from build123d import *

# Parameters (mm, degrees)
SKETCH1_R                 = 15.24
SKETCH1_R_2               = 6.35
BOSS_EXTRUDE1_DEPTH       = 6.35
F_4_CLEARANCE_HOLE1_D     = 2.9464
F_4_CLEARANCE_HOLE1_DEPTH = 6.35
BOSS_EXTRUDE2_DEPTH       = 6.35
CIRPATTERN1_COUNT         = 4


with BuildPart() as part:
    # Sketch1 → Boss-Extrude1 (new body)
    with BuildSketch(Plane(origin=(0, 0, 0), x_dir=(1, 0, 0), z_dir=(0, 1, 0))):
        Circle(SKETCH1_R)
        Circle(SKETCH1_R_2, mode=Mode.SUBTRACT)
    extrude(amount=BOSS_EXTRUDE1_DEPTH)

    # #4 Clearance Hole1
    with Locations(Plane(origin=(-8.015495471, 6.35, -5.066061758), x_dir=(1, 0, 0), z_dir=(0, 1, 0))):
        with Locations((8.015495471, 7.633938242), (-4.684504529, -5.066061758), (20.715495471, -5.066061758), (8.015495471, -17.766061758)):
            Hole(F_4_CLEARANCE_HOLE1_D / 2, depth=F_4_CLEARANCE_HOLE1_DEPTH)

    # Sketch7 → Boss-Extrude2 (add)
    with BuildSketch(Plane(origin=(0, 6.35, 0), x_dir=(1, 0, 0), z_dir=(0, 1, 0))):
        with BuildLine():
            ThreePointArc((-6.234328974, 13.9065), (0, 19.05), (6.234328974, 13.9065))
            ThreePointArc((6.234328974, 13.9065), (0, 15.24), (-6.234328974, 13.9065))
        make_face()
    boss_extrude2 = extrude(amount=-BOSS_EXTRUDE2_DEPTH)

    # CirPattern1: Boss-Extrude2 ×4 about axis
    cirpattern1_axis = Axis((0, 0, 0), (0, 1, 0))
    for i in range(1, CIRPATTERN1_COUNT):
        add(boss_extrude2.rotate(cirpattern1_axis, i * 360 / CIRPATTERN1_COUNT))


solid = part.part
Input: part model. Units: mm. Frame: model coordinates. Coordinates: 2 decimals unless noted, no trailing zeros. Order: outer loops, then holes, each group sorted by start corner. A loop starts at its lowest first (then second) coordinate and runs counter-clockwise, first axis right, second up. Notation, with made-up numbers: M 8.25,-15.5 L 45.25,-15.5 A23 cw 45.25,8.5 Z; hole C 59.5,-18 d2. An arc over 180 degrees is marked long. One line per question, with ' | ' between items.
Item 1: Pin query (flat end, axial travel): pin 1 (1.5 mm diameter, centred on x = -8, y = 5.5, fed in from -Z); pin 2 (1.8 mm diameter, centred on x = 12.7, z = 0, fed in from -Y). Return the tip coordinate at first contact, or that it passes through.
Geometry results:
pin 1: stops at z = -13.41 | pin 2: passes through
Item 2: Ray query, line 1 along Z through (x, y) = (3, 4); line 2 along X through (y, z) = (4.5, 12.7). Return the intervals inside material, ascending.
Geometry results:
line 1: z = -18.3 to -5.6, 5.6 to 18.3 | line 2: x = -8.42 to -1.47, 1.47 to 8.42
Item 3: Draft query along Z for faces 1 (the cylindrical face through (0.32, 3.13, -11.26)), 2 (the cylindrical face through (10.72, 3.13, 10.83)), 3 (the cylindrical face through (-19.05, 3.22, 0.12)). Return one class per face: released by +Z, released by -Z, zero draft, split by the parting line, or undercut.
Geometry results:
face 1: undercut | face 2: released by +Z | face 3: split by the parting line
Item 4: Section D-D (x = -12.7). Output: boundary loops of the cut face in (y, z), then the cut area to 3 significant figures.
Geometry results:
outline: M 0,-8.42 L 6.35,-8.42 L 6.35,-1.47 L 0,-1.47 Z; M 0,1.47 L 6.35,1.47 L 6.35,8.42 L 0,8.42 Z | area: 88.3 mm^2
Item 5: Section B-B (z = 0). Output: boundary loops of the cut face in (x, y), then the cut area to 3 significant figures.
Geometry results:
outline: M -19.05,0 L -14.17,0 L -14.17,6.35 L -19.05,6.35 Z; M -11.23,0 L -6.35,0 L -6.35,6.35 L -11.23,6.35 Z; M 6.35,0 L 11.23,0 L 11.23,6.35 L 6.35,6.35 Z; M 14.17,0 L 19.05,0 L 19.05,6.35 L 14.17,6.35 Z | area: 124 mm^2
Item 6: Section C-C (z = 4). Output: boundary loops of the cut face in (x, y), then the cut area to 3 significant figures.
Geometry results:
outline: M -17.63,0 L -4.93,0 L -4.93,6.35 L -17.63,6.35 Z; M 4.93,0 L 17.63,0 L 17.63,6.35 L 4.93,6.35 Z | area: 161 mm^2
Item 7: Section A-A (x = 0). Output: boundary loops of the cut face in (y, z).
Geometry results:
outline: M 0,-19.05 L 6.35,-19.05 L 6.35,-14.17 L 0,-14.17 Z; M 0,-11.23 L 6.35,-11.23 L 6.35,-6.35 L 0,-6.35 Z; M 0,6.35 L 6.35,6.35 L 6.35,11.23 L 0,11.23 Z; M 0,14.17 L 6.35,14.17 L 6.35,19.05 L 0,19.05 Z
